Autodesk Inventor part; units mm, degrees
ref_plane "C1_XY" through (0, 0, 0) normal (0, 0, 1) x (1, 0, 0)
ref_plane "C1_YZ" through (0, 0, 0) normal (1, 0, 0) x (0, 1, 0)
ref_plane "C1_ZX" through (0, 0, 0) normal (0, 1, 0) x (0, 0, 1)
sketch "Sketch_1" plane through (0, 0, 0) normal (0, 0, 1) x (1, 0, 0)
  line L0 (-10, -7) -> (-8, -7)
  line L1 (-8, -7) -> (-8, -4)
  line L2 (-8, -4) -> (-7.0607, -4)
  line L3 (-7.0607, -4) -> (-4, -7.0607)
  line L4 (-4, -7.0607) -> (-4, -9.4804)
  line L5 (-4, -9.4804) -> (-3.7, -10)
  line L6 (-3.7, -10) -> (-4, -10.5196)
  line L7 (-4, -10.5196) -> (-4, -12.9393)
  line L8 (-4, -12.9393) -> (-7.0607, -16)
  line L9 (-7.0607, -16) -> (-8, -16)
  line L10 (-8, -16) -> (-8, -13)
  line L11 (-8, -13) -> (-10, -13)
  line L12 (-10, -13) -> (-10, -19)
  arc A0 (-10, -19) -> (-9, -20) centre (-9, -19) ccw
  line L13 (-9, -20) -> (-3, -20)
  line L14 (-3, -20) -> (-3, -18)
  line L15 (-3, -18) -> (-6, -18)
  line L16 (-6, -18) -> (-6, -17.0607)
  line L17 (-6, -17.0607) -> (-2.9393, -14)
  line L18 (-2.9393, -14) -> (-0.5196, -14)
  line L19 (-0.5196, -14) -> (0, -13.7)
  line L20 (0, -13.7) -> (0.5196, -14)
  line L21 (0.5196, -14) -> (2.9393, -14)
  line L22 (2.9393, -14) -> (6, -17.0607)
  line L23 (6, -17.0607) -> (6, -18)
  line L24 (6, -18) -> (3, -18)
  line L25 (3, -18) -> (3, -20)
  line L26 (3, -20) -> (9, -20)
  arc A1 (9, -20) -> (10, -19) centre (9, -19) ccw
  line L27 (10, -19) -> (10, -13)
  line L28 (10, -13) -> (8, -13)
  line L29 (8, -13) -> (8, -16)
  line L30 (8, -16) -> (7.0607, -16)
  line L31 (7.0607, -16) -> (4, -12.9393)
  line L32 (4, -12.9393) -> (4, -10.5196)
  line L33 (4, -10.5196) -> (3.7, -10)
  line L34 (3.7, -10) -> (4, -9.4804)
  line L35 (4, -9.4804) -> (4, -7.0607)
  line L36 (4, -7.0607) -> (7.0607, -4)
  line L37 (7.0607, -4) -> (8, -4)
  line L38 (8, -4) -> (8, -7)
  line L39 (8, -7) -> (10, -7)
  line L40 (10, -7) -> (10, 7)
  line L41 (10, 7) -> (8, 7)
  line L42 (8, 7) -> (8, 4)
  line L43 (8, 4) -> (7.0607, 4)
  line L44 (7.0607, 4) -> (4, 7.0607)
  line L45 (4, 7.0607) -> (4, 9.4804)
  line L46 (4, 9.4804) -> (3.7, 10)
  line L47 (3.7, 10) -> (4, 10.5196)
  line L48 (4, 10.5196) -> (4, 12.9393)
  line L49 (4, 12.9393) -> (7.0607, 16)
  line L50 (7.0607, 16) -> (8, 16)
  line L51 (8, 16) -> (8, 13)
  line L52 (8, 13) -> (10, 13)
  line L53 (10, 13) -> (10, 19)
  arc A2 (10, 19) -> (9, 20) centre (9, 19) ccw
  line L54 (9, 20) -> (3, 20)
  line L55 (3, 20) -> (3, 18)
  line L56 (3, 18) -> (6, 18)
  line L57 (6, 18) -> (6, 17.0607)
  line L58 (6, 17.0607) -> (2.9393, 14)
  line L59 (2.9393, 14) -> (0.5196, 14)
  line L60 (0.5196, 14) -> (0, 13.7)
  line L61 (0, 13.7) -> (-0.5196, 14)
  line L62 (-0.5196, 14) -> (-2.9393, 14)
  line L63 (-2.9393, 14) -> (-6, 17.0607)
  line L64 (-6, 17.0607) -> (-6, 18)
  line L65 (-6, 18) -> (-3, 18)
  line L66 (-3, 18) -> (-3, 20)
  line L67 (-3, 20) -> (-9, 20)
  arc A3 (-9, 20) -> (-10, 19) centre (-9, 19) ccw
  line L68 (-10, 19) -> (-10, 13)
  line L69 (-10, 13) -> (-8, 13)
  line L70 (-8, 13) -> (-8, 16)
  line L71 (-8, 16) -> (-7.0607, 16)
  line L72 (-7.0607, 16) -> (-4, 12.9393)
  line L73 (-4, 12.9393) -> (-4, 10.5196)
  line L74 (-4, 10.5196) -> (-3.7, 10)
  line L75 (-3.7, 10) -> (-4, 9.4804)
  line L76 (-4, 9.4804) -> (-4, 7.0607)
  line L77 (-4, 7.0607) -> (-7.0607, 4)
  line L78 (-7.0607, 4) -> (-8, 4)
  line L79 (-8, 4) -> (-8, 7)
  line L80 (-8, 7) -> (-10, 7)
  line L81 (-10, 7) -> (-10, -7)
  line L82 (-8, 1.7) -> (-8, -1.7)
  arc A4 (-8, -1.7) -> (-7.7, -2) centre (-7.7, -1.7) ccw
  line L83 (-7.7, -2) -> (-7.0636, -2)
  arc A5 (-6.8515, -2.0879) -> (-7.0636, -2) centre (-7.0636, -2.3) ccw
  line L84 (-6.8515, -2.0879) -> (-2.9393, -6)
  line L85 (-2.9393, -6) -> (2.9393, -6)
  line L86 (2.9393, -6) -> (6.8515, -2.0879)
  arc A6 (7.0636, -2) -> (6.8515, -2.0879) centre (7.0636, -2.3) ccw
  line L87 (7.0636, -2) -> (7.7, -2)
  arc A7 (7.7, -2) -> (8, -1.7) centre (7.7, -1.7) ccw
  line L88 (8, -1.7) -> (8, 1.7)
  arc A8 (8, 1.7) -> (7.7, 2) centre (7.7, 1.7) ccw
  line L89 (7.7, 2) -> (7.0636, 2)
  arc A9 (6.8515, 2.0879) -> (7.0636, 2) centre (7.0636, 2.3) ccw
  line L90 (6.8515, 2.0879) -> (2.9393, 6)
  line L91 (2.9393, 6) -> (-2.9393, 6)
  line L92 (-2.9393, 6) -> (-6.8515, 2.0879)
  arc A10 (-7.0636, 2) -> (-6.8515, 2.0879) centre (-7.0636, 2.3) ccw
  line L93 (-7.0636, 2) -> (-7.7, 2)
  arc A11 (-7.7, 2) -> (-8, 1.7) centre (-7.7, 1.7) ccw
extrude "Extrusion1" add sketch "Sketch_1" against normal blind 350
sketch "Sketch2" plane through (0, 0, -350) normal (0, 0, -1) x (-1, 0, 0)
  point P0 (0, 10)
hole "Hole1" at (0, 10, -350) direction (0, 0, 1) diameter 4.2 depth 350
pattern_linear "Rectangular Pattern1" count 2 spacing 20 along (0, -1, 0) of "Hole1"
ref_plane "C1_XY" through (0, 0, 0) normal (0, 0, 1) x (1, 0, 0)
ref_plane "C1_YZ" through (0, 0, 0) normal (1, 0, 0) x (0, 1, 0)
ref_plane "C1_ZX" through (0, 0, 0) normal (0, 1, 0) x (0, 0, 1)
properties part number "HFS5-2040-350"
Geometry check sheet. Reference: the model listing, model coordinates, mm. A direction names the side the tool comes from. Give positions to 0.01 mm unless a question says otherwise; leave off trailing zeros. Use one line per item in the form item = value.
1) Material ranges on probe 1 along Y at (x, z) = (7.5, -245.5); probe 2 along Y at (x, z) = (0, -257); probe 3 along X at (y, z) = (-10, -113), recorded low to high. Write a range as from..to.
Working result:
probe_1 = -20..-16, -4..-2, 2..4, 16..20
probe_2 = -13.7..-12.1, -7.9..-6, 6..7.9, 12.1..13.7
probe_3 = -3.7..-2.1, 2.1..3.7
2) Draft check along Y on faces 3 (the face through (-10, 16, -173)), 4 (the face through (-6, 20, -173)), 5 (the face through (-6, -20, -173)), 6 (the face through (0, -6, -173)). Enter one of: released by +Y, released by -Y, zero draft, split by the parting line, or undercut.
Working result:
face_3 = zero draft
face_4 = released by +Y
face_5 = released by -Y
face_6 = undercut
3) Sectioned sample at A-A (z = -155.5). Count the separate pieces of the cut face and the enclosed holes in it, and give its area (3 significant figures).
Working result:
separate_pieces = 1
enclosed_holes = 3
area = 324 mm^2
4) Depth check by flat-ended pin: pin 1 Ø2 at (y, z) = (-10.5, -233) entering from +X; pin 2 Ø8 at (x, y) = (-7, 1) entering from -Z; pin 3 Ø3 at (x, z) = (0.5, -158) entering from +Y. Enter the tip coordinate at first touch or a pass-through.
Working result:
pin_1 = 4
pin_2 = -350
pin_3 = 14
5) Access from +Z, -Z, +X, -X, +Y, -Y to the whole of each face (thin tool, end or side, straight path). Record for faces 1 (the face through (-5, 5, 0)), 2 (the face through (0, 6, -173)).
Working result:
face_1 = +Z, +X, -X, +Y, -Y
face_2 = +Z, -Z
